Autodesk Inventor part; units mm, degrees
ref_plane "YZ Plane" through (0, 0, 0) normal (1, 0, 0) x (0, 1, 0)
ref_plane "XZ Plane" through (0, 0, 0) normal (0, 1, 0) x (-1, 0, 0)
ref_plane "XY Plane" through (0, 0, 0) normal (0, 0, 1) x (1, 0, 0)
sketch "스케치1" plane through (0, 0, 0) normal (0, 0, 1) x (1, 0, 0)
  line L0 (-60, -25) -> (60, -25)
  line L1 (60, -25) -> (60, 25)
  line L2 (60, 25) -> (-60, 25)
  line L3 (-60, 25) -> (-60, -25)
  line L4 (-60, -25) -> (60, 25) construction
  line L5 (60, -25) -> (-60, 25) construction
  point P0 (0, 0)
  dimension "d0" = 120
  dimension "d1" = 50
extrude "돌출1" add sketch "스케치1" along normal blind 3
sketch "스케치2" plane through (0, 0, 3) normal (0, 0, 1) x (1, 0, 0)
  line L0 (60, 25) -> (-60, 25)
  line L1 (60, 25) -> (57, 25)
  line L2 (57, 25) -> (57, 10)
  line L3 (57, 10) -> (60, 10)
  line L4 (60, 10) -> (60, 25)
  line L5 (-60, 0) -> (60, 0)
  line L6 (60, -25) -> (60, 25)
  line L7 (0, 25) -> (0, -25)
  line L8 (-60, -25) -> (60, -25)
  line L9 (60, -25) -> (57, -25)
  line L10 (57, -25) -> (57, -10)
  line L11 (57, -10) -> (60, -10)
  line L12 (60, -10) -> (60, -25)
  line L13 (-60, 25) -> (-57, 25)
  line L14 (-57, 25) -> (-57, 10)
  line L15 (-57, 10) -> (-60, 10)
  line L16 (-60, 10) -> (-60, 25)
  line L17 (-60, -25) -> (-57, -25)
  line L18 (-57, -25) -> (-57, -10)
  line L19 (-57, -10) -> (-60, -10)
  line L20 (-60, -10) -> (-60, -25)
  point P0 (0, 0)
  dimension "d4" = 3
  dimension "d5" = 15
extrude "돌출2" cut sketch "스케치2" against normal through all contours L4 L3 L2 L0 | L8 L20 L19 L18 | L14 L15 L16 L0 | L6 L8 L10 L11
sketch "스케치3" plane through (0, 0, 3) normal (0, 0, 1) x (1, 0, 0)
  line L0 (-15, 22) -> (15, 22)
  line L1 (15, 22) -> (15, 28)
  line L2 (15, 28) -> (-15, 28)
  line L3 (-15, 28) -> (-15, 22)
  line L4 (57, 25) -> (-57, 25)
  line L5 (-15, 22) -> (15, 28) construction
  line L6 (15, 22) -> (-15, 28) construction
  point P0 (0, 0)
  point P1 (0, 25)
  point P2 (15, 25)
  point P3 (-15, 25)
  dimension "d8" = 30
  dimension "d9" = 3
extrude "돌출3" cut sketch "스케치3" against normal through all contours L3 L4 L1 L0
sketch "스케치4" plane through (0, 0, 3) normal (0, 0, 1) x (1, 0, 0)
  line L0 (-15, -28) -> (15, -28)
  line L1 (15, -28) -> (15, -22)
  line L2 (15, -22) -> (-15, -22)
  line L3 (-15, -22) -> (-15, -28)
  line L4 (-57, -25) -> (57, -25)
  line L5 (-15, -28) -> (15, -22) construction
  line L6 (15, -28) -> (-15, -22) construction
  point P0 (0, 0)
  point P1 (0, -25)
  point P2 (15, -25)
  point P3 (-15, -25)
  dimension "d12" = 3
  dimension "d13" = 30
extrude "돌출4" add sketch "스케치4" against normal blind 3 contours L3 L4 L1 L0
sketch "스케치5" plane through (0, 0, 3) normal (0, 0, 1) x (1, 0, 0)
  circle A0 centre (-13.5, -10) radius 8.5
  circle A1 centre (13.5, -10) radius 8.5
  line L0 (15, -25) -> (57, -25)
  line L1 (-57, -25) -> (-15, -25)
  line L2 (60, -10) -> (60, 10)
  point P0 (0, 0)
  dimension "d16" = 27
  dimension "d18" = 17
  dimension "d19" = 17
  dimension "d22" = 15
  dimension "d23" = 15
  dimension "d24" = 46.5
extrude "돌출5" cut sketch "스케치5" against normal through all
sketch "스케치6" plane through (0, 0, 3) normal (0, 0, 1) x (1, 0, 0)
  point P0 (0, 0)
sketch "스케치7" plane through (0, 0, 3) normal (0, 0, 1) x (1, 0, 0)
  point P0 (0, 0)
properties part number "본체 겉면 레이저 앞판 수정"
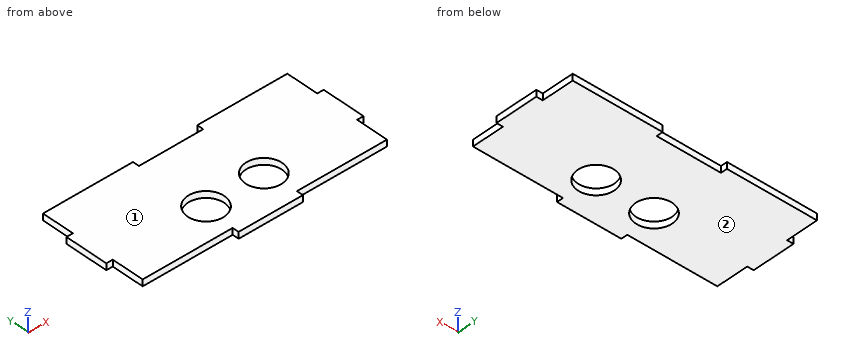
Geometry: final body of the model. Coordinates: model frame, mm. Face numbers are marked on the shaded views. Coordinates: 2 decimals unless noted, no trailing zeros. Order: outer loops, then holes, each group sorted by start corner. A loop starts at its lowest first (then second) coordinate and runs counter-clockwise, first axis right, second up. Notation, with made-up numbers: (-23.5, 72) - (26.5, 72) arc R10 cw to (26.5, 84) - close; hole circle Ø9 at (46.5, -24.75). An arc over 180 degrees is marked (long way). Return JSON: item names as keys, results as strings. Group by question number.
1. Cut plane A-A (z = 1.25). Output: boundary loops of the cut face in (x, y).
2. Pull-direction query (Z, two-part tool) for the marked faces 1 and 2; classes: pulls with the +Z half, pulls with the -Z half, needs draft (parallel to the pull), parting line crosses it, or undercut.
3. Cut plane D-D (x = -30.5). Output: boundary loops of the cut face in (y, z).
4. Material intervals for line 1 along Y through (x, z) = (13.5, 2.4); line 2 along X through (y, z) = (-15, 0.55); line 3 along X through (y, z) = (-14, 2.15), sorted ascending. Write a range as [from, to].
5. Cut plane C-C (y = -8). Output: boundary loops of the cut face in (x, z), plus the area to 3 significant figures.
6. Cut plane B-B (x = -13.5). Output: boundary loops of the cut face in (y, z), plus the area to 3 significant figures.
7. Pin query (flat end, axial travel): pin 1 (1.5 mm diameter, centred on y = 19.5, z = 2, fed in from -X); pin 2 (1.5 mm diameter, centred on x = -27.5, z = 1.5, fed in from -Y); pin 3 (1.5 mm diameter, centred on x = -4, z = 1.5, fed in from +Y); pin 4 (19.5 mm diameter, centred on x = 13.5, y = -10, fed in from -Z). Return the tip coordinate at first contact, or that it passes through.
Resolved:
{
 "1": {"outline": "(-60, -10) - (-57, -10) - (-57, -25) - (-15, -25) - (-15, -28) - (15, -28) - (15, -25) - (57, -25) - (57, -10) - (60, -10) - (60, 10) - (57, 10) - (57, 25) - (15, 25) - (15, 22) - (-15, 22) - (-15, 25) - (-57, 25) - (-57, 10) - (-60, 10) - close; hole circle Ø17 at (-13.5, -10); hole circle Ø17 at (13.5, -10)"},
 "2": {"face 1": "pulls with the +Z half", "face 2": "pulls with the -Z half"},
 "3": {"outline": "(-25, 0) - (25, 0) - (25, 3) - (-25, 3) - close"},
 "4": {"line 1": "y = [-28, -18.5], [-1.5, 22]", "line 2": "x = [-57, -20.37], [-6.63, 6.63], [20.37, 57]", "line 3": "x = [-57, -21], [-6, 6], [21, 57]"},
 "5": {"outline": "(-60, 0) - (-21.76, 0) - (-21.76, 3) - (-60, 3) - close; (-5.24, 0) - (5.24, 0) - (5.24, 3) - (-5.24, 3) - close; (21.76, 0) - (60, 0) - (60, 3) - (21.76, 3) - close", "area": "261 mm²"},
 "6": {"outline": "(-28, 0) - (-18.5, 0) - (-18.5, 3) - (-28, 3) - close; (-1.5, 0) - (22, 0) - (22, 3) - (-1.5, 3) - close", "area": "99.0 mm²"},
 "7": {"pin 1": "stops at x = -57", "pin 2": "stops at y = -25", "pin 3": "stops at y = 22", "pin 4": "stops at z = 0"}
}
